```python
from build123d import *

# Parameters (mm, degrees)
F1_DEPTH     = 99.822
F2_R         = 5.08
F3_R         = 5.08
F4_F1_R      = 5.08
F4_T2_DEPTH  = 89.662
F4_T7_DEPTH  = 5.1816
F4_T13_DEPTH = 5.1816
F4_T19_DEPTH = 5.1816
F4_T25_DEPTH = 5.1816
F4_T31_DEPTH = 5.1816
F4_T37_DEPTH = 5.1816
F4_T43_DEPTH = 5.1816
F4_T49_DEPTH = 5.1816
F4_T55_DEPTH = 5.1816
F4_T61_DEPTH = 5.1816


# Not quite as in the source:
# - a fillet or chamfer that OpenCascade refuses, or shapes differently, is made with other operations: its cross-section is extruded or revolved along the edge and cut away or added


with BuildPart() as f1:
    # F0 (on Right) → F1 (new body)
    with BuildSketch(Plane.YZ):
        Polygon((-82.3224335909, 15.9557517618), (-72.8414729238, 0), (122.7899119258, 0), (136.201992631, 39.3112748861), (40.6987294555, 62.4355487525), (7.1685267612, 58.7356649339), (-27.5178905576, 39.3112748861), (-67.0604035258, 31.9115035236), align=None)
    extrude(amount=F1_DEPTH)

    # F2
    f2_edges = [f1.edges().sort_by_distance(p)[0] for p in [
        (99.822, -47.289147, 35.611389),
        (99.822, -74.691419, 23.933628),
        (99.822, -77.581953, 7.977876),
        (99.822, 24.97422, 0),
        (99.822, 129.495952, 19.655637),
        (99.822, 88.450361, 50.873412),
        (99.822, 23.933628, 60.585607),
        (99.822, -10.174682, 49.02347),
    ]]
    fillet(f2_edges, radius=F2_R)

    # F3
    f3_edges = [f1.edges().sort_by_distance(p)[0] for p in [
        (0, -47.289147, 35.611389),
        (0, -74.691419, 23.933628),
        (0, -77.581953, 7.977876),
        (0, 24.97422, 0),
        (0, 129.495952, 19.655637),
        (0, 88.450361, 50.873412),
        (0, 23.933628, 60.585607),
        (0, -10.174682, 49.02347),
    ]]
    fillet(f3_edges, radius=F3_R)

    # F4: fillet of radius 5.08 on 8 edges, made by hand

    # F4_f1
    f4_f1_edges = [f1.edges().sort_by_distance(p)[0] for p in [
        (49.911, -27.5178905576, 39.3112748861),
        (1.4878975516, -27.0040618743, 37.8937040228),
        (98.3341025696, -27.0040618325, 37.8937039074),
    ]]
    fillet(f4_f1_edges, radius=F4_F1_R)

    # F4_s3 → F4_t2 (cut)
    with BuildSketch(Plane.YZ.offset(5.08)):
        with BuildLine():
            ThreePointArc((-65.453685614, 32.2121759973), (-66.9382582043, 31.6859414336), (-68.1902824988, 30.7302669295))
            Line((-68.1902824988, 30.7302669295), (-68.2637028962, 30.8004951663))
            Line((-68.2637028962, 30.8004951663), (-67.1112263438, 32.0053564923))
            Line((-67.1112263438, 32.0053564923), (-65.4723740737, 32.3120424155))
            Line((-65.4723740737, 32.3120424155), (-65.453685614, 32.2121759973))
        make_face()
        with BuildLine():
            ThreePointArc((-79.6549091873, 18.7445260612), (-81.0311938802, 15.8085415748), (-80.3510820874, 12.6381137788))
            Line((-80.3510820874, 12.6381137788), (-80.4384259429, 12.5862137699))
            Line((-80.4384259429, 12.5862137699), (-82.4492044764, 15.9702045126))
            Line((-82.4492044764, 15.9702045126), (-79.7283295848, 18.8147542979))
            Line((-79.7283295848, 18.8147542979), (-79.6549091873, 18.7445260612))
        make_face()
        with BuildLine():
            ThreePointArc((6.2686920086, 58.2317575672), (7.2001593092, 58.6369802666), (8.1936269176, 58.8487794151))
            Line((8.1936269176, 58.8487794151), (8.1824835206, 58.9497664672))
            Line((8.1824835206, 58.9497664672), (7.1368813611, 58.8343896965))
            Line((7.1368813611, 58.8343896965), (6.2190499134, 58.3204041823))
            Line((6.2190499134, 58.3204041823), (6.2686920086, 58.2317575672))
        make_face()
        with BuildLine():
            ThreePointArc((39.8125749839, 62.3377662065), (40.6937772364, 62.3580687153), (41.5652241428, 62.2257437701))
            Line((41.5652241428, 62.2257437701), (41.589133729, 62.3244903735))
            Line((41.589133729, 62.3244903735), (40.7053091479, 62.5384914556))
            Line((40.7053091479, 62.5384914556), (39.8014315869, 62.4387532586))
            Line((39.8014315869, 62.4387532586), (39.8125749839, 62.3377662065))
        make_face()
        with BuildLine():
            ThreePointArc((130.792336403, 40.6211188431), (134.0495526612, 38.1291725243), (134.4047361425, 34.0434536277))
            Line((134.4047361425, 34.0434536277), (134.5008937235, 34.0106469268))
            Line((134.5008937235, 34.0106469268), (136.3340953417, 39.3838246104))
            Line((136.3340953417, 39.3838246104), (130.8162459892, 40.7198654465))
            Line((130.8162459892, 40.7198654465), (130.792336403, 40.6211188431))
        make_face()
    extrude(amount=F4_T2_DEPTH, mode=Mode.SUBTRACT)


with BuildPart() as f4_tool5:
    # F4_s6 → F4_t7 (new body)
    with BuildSketch(Plane.YZ.offset(5.08)):
        Polygon((129.5968570941, 35.6837886716), (130.8162459892, 40.7198654465), (136.3340953417, 39.3838246104), (134.5008937235, 34.0106469268), align=None)
    extrude(amount=-F4_T7_DEPTH)

    # F4_s8 → F4_t9 (revolve, cut)
    with BuildSketch(Plane(origin=(5.08, 129.5968570941, 35.6837886716), x_dir=(0, -0.8765148754, -0.4813747742), z_dir=(0, 0.4813747742, -0.8765148754))):
        with BuildLine():
            ThreePointArc((0, -5.08), (5.08, 0), (0, 5.08))
            Line((0, 5.08), (0, -5.08))
        make_face()
    revolve(axis=Axis((5.08, 129.5968570941, 35.6837886716), (-1, 0, 0)), mode=Mode.SUBTRACT)


with BuildPart() as f1_1:
    add(f1.part)

    # F4_t4: cut F4_tool5
    add(f4_tool5.part, mode=Mode.SUBTRACT)


with BuildPart() as f4_tool11:
    # F4_s12 → F4_t13 (new body)
    with BuildSketch(Plane.YZ.offset(94.742)):
        Polygon((129.5968570941, 35.6837886716), (130.8162459892, 40.7198654465), (136.3340953417, 39.3838246104), (134.5008937235, 34.0106469268), align=None)
    extrude(amount=F4_T13_DEPTH)

    # F4_s14 → F4_t15 (revolve, cut)
    with BuildSketch(Plane(origin=(94.742, 129.5968570941, 35.6837886716), x_dir=(0, -0.8765148754, -0.4813747742), z_dir=(0, -0.4813747742, 0.8765148754))):
        with BuildLine():
            ThreePointArc((0, -5.08), (5.08, 0), (0, 5.08))
            Line((0, 5.08), (0, -5.08))
        make_face()
    revolve(axis=Axis((94.742, 129.5968570941, 35.6837886716), (1, 0, 0)), mode=Mode.SUBTRACT)


with BuildPart() as f1_2:
    add(f1_1.part)

    # F4_t10: cut F4_tool11
    add(f4_tool11.part, mode=Mode.SUBTRACT)


with BuildPart() as f4_tool17:
    # F4_s18 → F4_t19 (new body)
    with BuildSketch(Plane.YZ.offset(5.08)):
        Polygon((40.369744834, 57.2884135986), (39.8014315869, 62.4387532586), (40.7053091479, 62.5384914556), (41.589133729, 62.3244903735), align=None)
    extrude(amount=-F4_T19_DEPTH)

    # F4_s20 → F4_t21 (revolve, cut)
    with BuildSketch(Plane(origin=(5.08, 40.369744834, 57.2884135986), x_dir=(0, -0.063785906, -0.9979636056), z_dir=(0, 0.9979636056, -0.063785906))):
        with BuildLine():
            ThreePointArc((0, -5.08), (5.08, 0), (0, 5.08))
            Line((0, 5.08), (0, -5.08))
        make_face()
    revolve(axis=Axis((5.08, 40.369744834, 57.2884135986), (-1, 0, 0)), mode=Mode.SUBTRACT)


with BuildPart() as f1_3:
    add(f1_2.part)

    # F4_t16: cut F4_tool17
    add(f4_tool17.part, mode=Mode.SUBTRACT)


with BuildPart() as f4_tool23:
    # F4_s24 → F4_t25 (new body)
    with BuildSketch(Plane.YZ.offset(94.742)):
        Polygon((40.369744834, 57.2884135986), (39.8014315869, 62.4387532586), (40.7053091479, 62.5384914556), (41.589133729, 62.3244903735), align=None)
    extrude(amount=F4_T25_DEPTH)

    # F4_s26 → F4_t27 (revolve, cut)
    with BuildSketch(Plane(origin=(94.742, 40.369744834, 57.2884135986), x_dir=(0, -0.063785906, -0.9979636056), z_dir=(0, -0.9979636056, 0.063785906))):
        with BuildLine():
            ThreePointArc((0, -5.08), (5.08, 0), (0, 5.08))
            Line((0, 5.08), (0, -5.08))
        make_face()
    revolve(axis=Axis((94.742, 40.369744834, 57.2884135986), (1, 0, 0)), mode=Mode.SUBTRACT)


with BuildPart() as f1_4:
    add(f1_3.part)

    # F4_t22: cut F4_tool23
    add(f4_tool23.part, mode=Mode.SUBTRACT)


with BuildPart() as f4_tool29:
    # F4_s30 → F4_t31 (new body)
    with BuildSketch(Plane.YZ.offset(5.08)):
        Polygon((8.7507967676, 53.7994268073), (6.2190499134, 58.3204041823), (7.1368813611, 58.8343896965), (8.1824835206, 58.9497664672), align=None)
    extrude(amount=-F4_T31_DEPTH)

    # F4_s32 → F4_t33 (revolve, cut)
    with BuildSketch(Plane(origin=(5.08, 8.7507967676, 53.7994268073), x_dir=(0, 0.3052435942, -0.952274303), z_dir=(0, 0.952274303, 0.3052435942))):
        with BuildLine():
            ThreePointArc((0, -5.08), (5.08, 0), (0, 5.08))
            Line((0, 5.08), (0, -5.08))
        make_face()
    revolve(axis=Axis((5.08, 8.7507967676, 53.7994268073), (-1, 0, 0)), mode=Mode.SUBTRACT)


with BuildPart() as f1_5:
    add(f1_4.part)

    # F4_t28: cut F4_tool29
    add(f4_tool29.part, mode=Mode.SUBTRACT)


with BuildPart() as f4_tool35:
    # F4_s36 → F4_t37 (new body)
    with BuildSketch(Plane.YZ.offset(94.742)):
        Polygon((8.7507967676, 53.7994268073), (6.2190499134, 58.3204041823), (7.1368813611, 58.8343896965), (8.1824835206, 58.9497664672), align=None)
    extrude(amount=F4_T37_DEPTH)

    # F4_s38 → F4_t39 (revolve, cut)
    with BuildSketch(Plane(origin=(94.742, 8.7507967676, 53.7994268073), x_dir=(0, 0.3052435942, -0.952274303), z_dir=(0, -0.952274303, -0.3052435942))):
        with BuildLine():
            ThreePointArc((0, -5.08), (5.08, 0), (0, 5.08))
            Line((0, 5.08), (0, -5.08))
        make_face()
    revolve(axis=Axis((94.742, 8.7507967676, 53.7994268073), (1, 0, 0)), mode=Mode.SUBTRACT)


with BuildPart() as f1_6:
    add(f1_5.part)

    # F4_t34: cut F4_tool35
    add(f4_tool35.part, mode=Mode.SUBTRACT)


with BuildPart() as f4_tool41:
    # F4_s42 → F4_t43 (new body)
    with BuildSketch(Plane.YZ.offset(5.08)):
        Polygon((-75.9838893162, 15.2331142218), (-79.7283295848, 18.8147542979), (-82.4492044764, 15.9702045126), (-80.4384259429, 12.5862137699), align=None)
    extrude(amount=-F4_T43_DEPTH)

    # F4_s44 → F4_t45 (revolve, cut)
    with BuildSketch(Plane(origin=(5.08, -75.9838893162, 15.2331142218), x_dir=(0, 0.9935638905, -0.113273101), z_dir=(0, 0.113273101, 0.9935638905))):
        with BuildLine():
            ThreePointArc((0, -5.08), (5.08, 0), (0, 5.08))
            Line((0, 5.08), (0, -5.08))
        make_face()
    revolve(axis=Axis((5.08, -75.9838893162, 15.2331142218), (-1, 0, 0)), mode=Mode.SUBTRACT)


with BuildPart() as f1_7:
    add(f1_6.part)

    # F4_t40: cut F4_tool41
    add(f4_tool41.part, mode=Mode.SUBTRACT)


with BuildPart() as f4_tool47:
    # F4_s48 → F4_t49 (new body)
    with BuildSketch(Plane.YZ.offset(94.742)):
        Polygon((-75.9838893162, 15.2331142218), (-79.7283295848, 18.8147542979), (-82.4492044764, 15.9702045126), (-80.4384259429, 12.5862137699), align=None)
    extrude(amount=F4_T49_DEPTH)

    # F4_s50 → F4_t51 (revolve, cut)
    with BuildSketch(Plane(origin=(94.742, -75.9838893162, 15.2331142218), x_dir=(0, 0.9935638905, -0.113273101), z_dir=(0, -0.113273101, -0.9935638905))):
        with BuildLine():
            ThreePointArc((0, -5.08), (5.08, 0), (0, 5.08))
            Line((0, 5.08), (0, -5.08))
        make_face()
    revolve(axis=Axis((94.742, -75.9838893162, 15.2331142218), (1, 0, 0)), mode=Mode.SUBTRACT)


with BuildPart() as f1_8:
    add(f1_7.part)

    # F4_t46: cut F4_tool47
    add(f4_tool47.part, mode=Mode.SUBTRACT)


with BuildPart() as f4_tool53:
    # F4_s54 → F4_t55 (new body)
    with BuildSketch(Plane.YZ.offset(5.08)):
        Polygon((-64.5192626277, 27.2188550901), (-65.4723740737, 32.3120424155), (-67.1112263438, 32.0053564923), (-68.2637028962, 30.8004951663), align=None)
    extrude(amount=-F4_T55_DEPTH)

    # F4_s56 → F4_t57 (revolve, cut)
    with BuildSketch(Plane(origin=(5.08, -64.5192626277, 27.2188550901), x_dir=(0, 0.4761802316, -0.8793477054), z_dir=(0, 0.8793477054, 0.4761802316))):
        with BuildLine():
            ThreePointArc((0, -5.08), (5.08, 0), (0, 5.08))
            Line((0, 5.08), (0, -5.08))
        make_face()
    revolve(axis=Axis((5.08, -64.5192626277, 27.2188550901), (-1, 0, 0)), mode=Mode.SUBTRACT)


with BuildPart() as f1_9:
    add(f1_8.part)

    # F4_t52: cut F4_tool53
    add(f4_tool53.part, mode=Mode.SUBTRACT)


with BuildPart() as f4_tool59:
    # F4_s60 → F4_t61 (new body)
    with BuildSketch(Plane.YZ.offset(94.742)):
        Polygon((-64.5192626277, 27.2188550901), (-65.4723740737, 32.3120424155), (-67.1112263438, 32.0053564923), (-68.2637028962, 30.8004951663), align=None)
    extrude(amount=F4_T61_DEPTH)

    # F4_s62 → F4_t63 (revolve, cut)
    with BuildSketch(Plane(origin=(94.742, -64.5192626277, 27.2188550901), x_dir=(0, 0.4761802316, -0.8793477054), z_dir=(0, -0.8793477054, -0.4761802316))):
        with BuildLine():
            ThreePointArc((0, -5.08), (5.08, 0), (0, 5.08))
            Line((0, 5.08), (0, -5.08))
        make_face()
    revolve(axis=Axis((94.742, -64.5192626277, 27.2188550901), (1, 0, 0)), mode=Mode.SUBTRACT)


with BuildPart() as f1_10:
    add(f1_9.part)

    # F4_t58: cut F4_tool59
    add(f4_tool59.part, mode=Mode.SUBTRACT)


solid = f1_10.part
```
For this review, take the finished solid that the model builds, in its own axes (mm). Coordinates: 2 decimals unless noted, no trailing zeros. Loops run counter-clockwise (first coordinate to the right, second up) from the corner with the lowest first, then second, coordinate; pieces in that order, holes last.
1. Add section A-A, the plane x = 52. Give the boundary of the cut face in (y, z), then the cut area to 3 significant figures.
2. For line 1 (Z direction, x = 40, y = -33); line 2 (Z direction, x = 45.5, y = 110.5); line 3 (Y direction, x = 32.5, z = 40), list the stretches that pass through material, from the lowest coordinate up.
3. Insertion check: P1, Ø10, axis at x = 77.5, z = 43, coming from the +Y side; P2, Ø3, axis at x = 78.5, z = 41.5, coming from the +Y side; P3, Ø1.5, axis at x = 19.5, z = 16.5, coming from the +Y side. Each pin has a flat end and moves straight along its axis. Give the tip position at first contact, or say it passes through.
Result:
1. outline: (-80.35, 12.64) - (-72.84, 0) - (122.79, 0) - (134.4, 34.04) arc R5.08 ccw to (130.79, 40.62) - (41.57, 62.23) arc R5.08 ccw to (39.81, 62.34) - (8.19, 58.85) arc R5.08 ccw to (6.27, 58.23) - (-26.79, 39.72) arc R5.08 cw to (-28.34, 39.16) - (-65.45, 32.21) arc R5.08 ccw to (-68.19, 30.73) - (-79.65, 18.74) arc R5.08 ccw to start
1. area: 10,000 mm2
2. line 1: z = 0 to 38.29
2. line 2: z = 0 to 45.53
2. line 3: y = -26.29 to 132.28
3. P1: stops at y = 134.12
3. P2: stops at y = 132.28
3. P3: stops at y = 128.68
